Verification items for this drawing (mm, ordinates from the low corner). Round coordinates to 2 decimals unless told otherwise and drop trailing zeros. Order: outer loops, then holes, each group sorted by start corner. A loop starts at its lowest first (then second) coordinate and runs counter-clockwise, first axis right, second up. Notation, with made-up numbers: (55.5, 69) -> (59.5, 69) arc R29 cw to (59.5, 96) -> close; hole circle Ø8 at (-34, 3). An arc over 180 degrees is marked (long way). Answer in a Markdown table with one row per item.
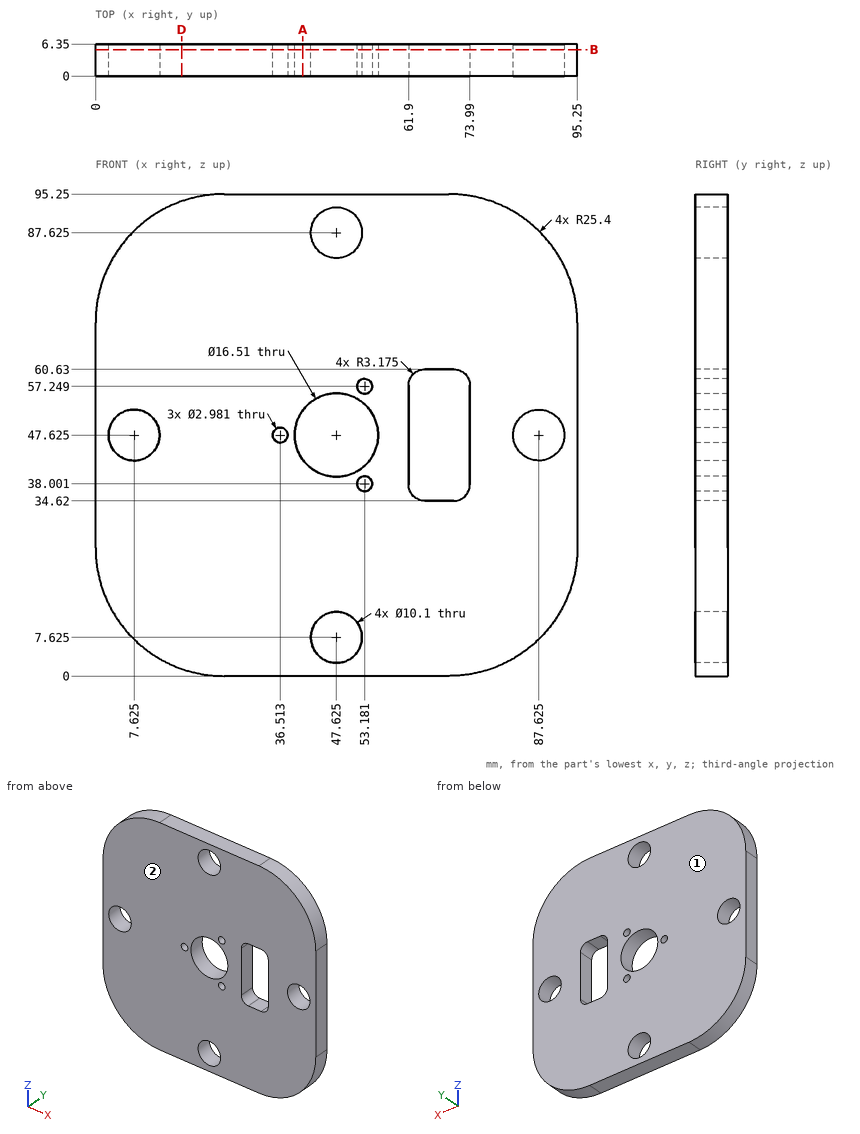
Item 1: Cross-section at A-A (x = 41). Record the boundary of the cut face in (y, z).
Result sheet:
| item | result |
|---|---|
| outline | (0, 0) -> (6.35, 0) -> (6.35, 42.7) -> (0, 42.7) -> close; (0, 52.55) -> (6.35, 52.55) -> (6.35, 95.25) -> (0, 95.25) -> close |
Item 2: Depth check by flat-ended pin: P1, Ø1, axis at y = 2, z = 70.5, coming from the +X side; P2, Ø9, axis at x = 87.625, z = 47.625, coming from the +Y side; P3, Ø1.5, axis at x = 14, y = 4, coming from the +Z side. Enter the tip coordinate at first touch or a pass-through.
Result sheet:
| item | result |
|---|---|
| P1 | stops at x = 95.25 |
| P2 | passes through |
| P3 | stops at z = 92.91 |
Item 3: Mould release check, pull along Y, two halves, no side actions. Record for the marked faces 1 and 2: pulls with the +Y half, pulls with the -Y half, needs draft (parallel to the pull), parting line crosses it, or undercut.
Result sheet:
| item | result |
|---|---|
| face 1 | pulls with the +Y half |
| face 2 | pulls with the -Y half |
Item 4: Cross-section at B-B (y = 5.25). State how many separate pieces and enclosed holes the cut face has, and give its area (3 significant figures).
Result sheet:
| item | result |
|---|---|
| separate pieces | 1 |
| enclosed holes | 9 |
| area | 7,660 mm^2 |
Item 5: Cross-section at D-D (x = 17). Record the boundary of the cut face in (y, z).
Result sheet:
| item | result |
|---|---|
| outline | (0, 1.43) -> (6.35, 1.43) -> (6.35, 93.82) -> (0, 93.82) -> close |
Item 6: Scan lines: line 1 (X direction, y = 4.25, z = 57); line 2 (X direction, y = 3, z = 56.5); line 3 (Z direction, x = 48.5, y = 0.5). Record each from-to range of solid material in increasing order. Write a range as [from, to].
Result sheet:
| item | result |
|---|---|
| line 1 | x = [0, 51.71], [54.65, 61.9], [73.99, 95.25] |
| line 2 | x = [0, 51.89], [54.47, 61.9], [73.99, 95.25] |
| line 3 | z = [0, 2.65], [12.6, 39.42], [55.83, 82.65], [92.6, 95.25] |
